Autodesk Inventor part; units mm, degrees
ref_plane "YZ Plane" through (0, 0, 0) normal (1, 0, 0) x (0, 1, 0)
ref_plane "XZ Plane" through (0, 0, 0) normal (0, 1, 0) x (-1, 0, 0)
ref_plane "XY Plane" through (0, 0, 0) normal (0, 0, 1) x (1, 0, 0)
sketch "Sketch1" plane through (0, 0, 0) normal (0, 0, 1) x (1, 0, 0)
  line L0 (0, 0) -> (0, 20) construction
  line L1 (0, 20) -> (-4, 20)
  line L2 (-4, 0) -> (-4, 20)
  line L3 (0, 0) -> (-4, 0)
  line L4 (0, 40) -> (0, 60) construction
  line L5 (0, 60) -> (-4, 60)
  line L6 (-4, 40) -> (-4, 60)
  line L7 (0, 40) -> (-4, 40)
  line L8 (0, 70) -> (-4, 70) construction
  line L9 (0, 70) -> (80, 70)
  line L10 (80, 70) -> (80, 60)
  line L11 (80, -10) -> (0, -10) construction
  line L12 (0, -10) -> (0, 0)
  line L13 (40, 70) -> (40, -10) construction
  line L14 (0, 60) -> (0, 70)
  line L15 (0, 40) -> (0, 60) construction
  line L16 (0, 20) -> (0, 40)
  line L17 (0, 0) -> (0, 20) construction
  line L18 (80, 20) -> (84, 20)
  line L19 (84, 0) -> (84, 20)
  line L20 (80, 0) -> (84, 0)
  line L21 (80, 60) -> (84, 60)
  line L22 (84, 40) -> (84, 60)
  line L23 (80, 40) -> (84, 40)
  line L24 (80, 70) -> (84, 70) construction
  line L25 (80, 60) -> (80, 40) construction
  line L26 (80, 40) -> (80, 20)
  line L27 (80, 20) -> (80, 0) construction
  line L28 (80, 0) -> (80, -10)
  line L29 (10, -10) -> (10, -14)
  line L30 (10, -14) -> (30, -14)
  line L31 (30, -10) -> (30, -14)
  line L32 (50, -10) -> (50, -14)
  line L33 (50, -14) -> (70, -14)
  line L34 (70, -10) -> (70, -14)
  line L35 (10, -10) -> (0, -10)
  line L36 (30, -10) -> (50, -10)
  line L37 (70, -10) -> (80, -10)
  point P0 (40, 30)
  dimension "d0" = 80
  dimension "d1" = 80
  dimension "d6" = 90
extrude "Extrusion1" add sketch "Sketch1" along normal blind 4
sketch "Sketch2" plane through (0, 0, 4) normal (0, 0, 1) x (1, 0, 0)
  line L0 (0, 20) -> (-4, 20) construction
  line L1 (-4, 20) -> (-4, 0) construction
  line L2 (-4, 0) -> (0, 0) construction
  line L3 (0, 0) -> (0, -10) construction
  line L4 (0, -10) -> (10, -10) construction
  line L5 (10, -10) -> (10, -14) construction
  line L6 (10, -14) -> (30, -14) construction
  line L7 (30, -14) -> (30, -10) construction
  line L8 (30, -10) -> (50, -10) construction
  line L9 (50, -10) -> (50, -14) construction
  line L10 (50, -14) -> (70, -14) construction
  line L11 (70, -14) -> (70, -10) construction
  line L12 (70, -10) -> (80, -10) construction
  line L13 (80, -10) -> (80, 0) construction
  line L14 (80, 0) -> (84, 0) construction
  line L15 (84, 0) -> (84, 20) construction
  line L16 (84, 20) -> (80, 20) construction
  line L17 (80, 20) -> (80, 40) construction
  line L18 (80, 40) -> (84, 40) construction
  line L19 (84, 40) -> (84, 60) construction
  line L20 (84, 60) -> (80, 60) construction
  line L21 (80, 60) -> (80, 70) construction
  line L22 (80, 70) -> (0, 70) construction
  line L23 (0, 70) -> (0, 60) construction
  line L24 (0, 60) -> (-4, 60) construction
  line L25 (-4, 60) -> (-4, 40) construction
  line L26 (-4, 40) -> (0, 40) construction
  line L27 (0, 40) -> (0, 20) construction
  line L28 (0, 31.5) -> (12, 31.5)
  line L29 (12, 31.5) -> (12, 28.5)
  line L30 (12, 28.5) -> (0, 28.5)
  line L31 (0, 28.5) -> (0, 31.5)
  line L32 (80, 28.5) -> (68, 28.5)
  line L33 (68, 28.5) -> (68, 31.5)
  line L34 (68, 31.5) -> (80, 31.5)
  line L35 (80, 31.5) -> (80, 28.5)
  line L36 (0, 40) -> (0, 20)
  line L37 (4.8, 32.7) -> (7.2, 32.7)
  line L38 (7.2, 32.7) -> (7.2, 27.3)
  line L39 (7.2, 27.3) -> (4.8, 27.3)
  line L40 (4.8, 27.3) -> (4.8, 32.7)
  line L41 (72.8, 32.7) -> (75.2, 32.7)
  line L42 (75.2, 32.7) -> (75.2, 27.3)
  line L43 (75.2, 27.3) -> (72.8, 27.3)
  line L44 (72.8, 27.3) -> (72.8, 32.7)
  line L45 (38.5, -10) -> (41.5, -10)
  line L46 (41.5, -10) -> (41.5, 2)
  line L47 (41.5, 2) -> (38.5, 2)
  line L48 (38.5, 2) -> (38.5, -10)
  line L49 (37.3, -5.2) -> (42.7, -5.2)
  line L50 (42.7, -5.2) -> (42.7, -2.8)
  line L51 (42.7, -2.8) -> (37.3, -2.8)
  line L52 (37.3, -2.8) -> (37.3, -5.2)
  line L53 (30, -10) -> (50, -10)
  point P0 (7.2, 30)
  point P1 (72.8, 30)
  point P2 (68, 30)
  point P3 (12, 30)
  point P4 (6, 32.7)
  point P5 (6, 31.5)
  point P6 (74, 32.7)
  point P7 (74, 31.5)
  point P8 (0, 30)
  point P9 (0, 30)
  point P10 (37.3, -4)
  point P11 (38.5, -4)
  point P12 (40, -2.8)
  point P13 (40, 2)
  point P14 (40, -10)
  point P15 (40, -10)
  point P16 (40, -10)
  point P17 (4.8, 31.5)
  point P18 (4.8, 28.5)
  point P19 (7.2, 28.5)
  point P20 (7.2, 31.5)
  point P21 (38.5, -5.2)
  point P22 (41.5, -5.2)
  point P23 (41.5, -2.8)
  point P24 (38.5, -2.8)
  point P25 (72.8, 28.5)
  point P26 (75.2, 28.5)
  point P27 (75.2, 31.5)
  point P28 (72.8, 31.5)
  dimension "d8" = 2.4
  dimension "d9" = 5.4
  dimension "d10" = 3
  dimension "d11" = 12
extrude "Extrusion2" cut sketch "Sketch2" against normal up to next
properties part number "Car_Left" material "MDF Medium Density Fiberboard"
Model file for the job. Use its own axes, mm. A direction names the side the tool comes from. Coordinates: 2 decimals unless noted, no trailing zeros. Order: outer loops, then holes, each group sorted by start corner. A loop starts at its lowest first (then second) coordinate and runs counter-clockwise, first axis right, second up. Notation, with made-up numbers: (72.25, 62.5) -> (104.25, 62.5) arc R17 cw to (104.25, 71.5) -> close; hole circle Ø6 at (13.5, 3). An arc over 180 degrees is marked (long way). Return JSON: item names as keys, results as strings.
Item 1: Wall check: line 1 along Y through (x, z) = (69, 2.1); line 2 along X through (y, z) = (-7.5, 2.15); line 3 along X through (y, z) = (63.5, 3.5). Give the ranges that are in metal, low to high. Write a range as from..to.
Model answer:
{"line 1": "y = -14..28.5, 31.5..70", "line 2": "x = 0..38.5, 41.5..80", "line 3": "x = 0..80"}
Item 2: Slice it at B-B (y = 22.5). Write the cut outline in (x, z), then the cut area to 3 significant figures.
Model answer:
{"outline": "(0, 0) -> (80, 0) -> (80, 4) -> (0, 4) -> close", "area": "320 mm²"}
Item 3: 3-axis set-ups, long thin cutter, end or side, ignore diameter. For faces 1 (the face through (10, -12, 2)), 2 (the face through (70, 28.5, 2)), 3 (the face through (-2, 60, 2)), 4 (the face through (50, -12, 2)): which of +Z, -Z, +X, -X, +Y, -Y reach the whole face in a straight line?
Model answer:
{"face 1": "+Z, -Z, -X, -Y", "face 2": "+Z, -Z, +X", "face 3": "+Z, -Z, -X, +Y", "face 4": "+Z, -Z, -Y"}
Item 4: Slice it at A-A (x = 45). Write the cut outline in (y, z).
Model answer:
{"outline": "(-10, 0) -> (70, 0) -> (70, 4) -> (-10, 4) -> close"}
Item 5: Pin check, flat tips, straight feed: P1, Ø1, axis at y = 26.5, z = 2.5, coming from the +X side; P2, Ø1.9, axis at x = 6, z = 2.5, coming from the -Y side; P3, Ø2, axis at y = -12.5, z = 2.5, coming from the +X side. Stop position of each tip, or through.
Model answer:
{"P1": "stops at x = 80", "P2": "stops at y = -10", "P3": "stops at x = 70"}
Item 6: Mould opens along X. For faces 5 (the face through (74, 32.7, 2)), 6 (the face through (0, 65, 2)), 7 (the face through (-2, 0, 2)), 8 (the face through (6, 32.7, 2)) say: pulls with the +X half, pulls with the -X half, needs draft (parallel to the pull), parting line crosses it, or undercut.
Model answer:
{"face 5": "undercut", "face 6": "pulls with the -X half", "face 7": "needs draft", "face 8": "undercut"}
